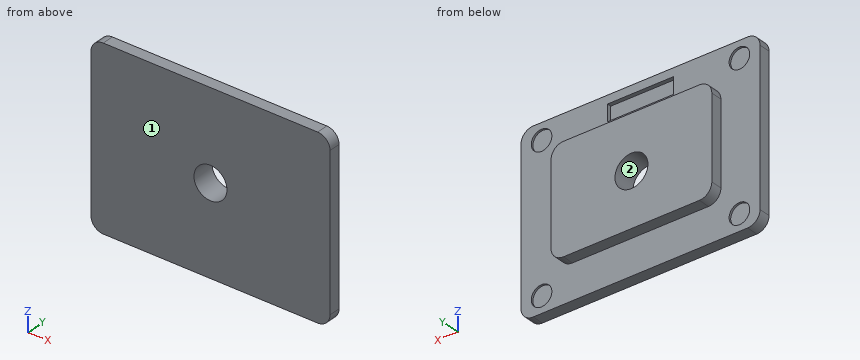
```python
from build123d import *

# Parameters (mm, degrees)
SKETCH3_W                      = 73.66
SKETCH3_H                      = 54.61
EXTRUDED_LOWER_PLATE_DEPTH     = 3.556
SKETCH4_W                      = 49.53
SKETCH4_H                      = 33.02
EXTRUDED_UPPER_PLATE_DEPTH     = 3.556
PLATE_CORNER_FILLET_R          = 3.81
F_0_4D_HOLE_D                  = 10.16
SKETCH9_W                      = 20.32
SKETCH9_H                      = 5.08
EXTRUDED_RECTANGULAR_CUT_DEPTH = 1.27
F_4X_0_25D_PINS_D              = 6.35
F_4X_0_25D_PINS_DEPTH          = 0.635


with BuildPart() as part:
    # Sketch3 → Extruded Lower Plate (new body)
    with BuildSketch(Plane(origin=(0, 0, 0), x_dir=(1, 0, 0), z_dir=(0, 1, 0))):
        Rectangle(SKETCH3_W, SKETCH3_H)
    extrude(amount=EXTRUDED_LOWER_PLATE_DEPTH)

    # Sketch4 → Extruded Upper Plate (add)
    with BuildSketch(Plane(origin=(0, 3.556, 0), x_dir=(1, 0, 0), z_dir=(0, 1, 0))):
        Rectangle(SKETCH4_W, SKETCH4_H)
    extrude(amount=EXTRUDED_UPPER_PLATE_DEPTH)

    # Plate Corner Fillet
    plate_corner_fillet_edges = [part.edges().sort_by_distance(p)[0] for p in [
        (24.765, 5.334, -16.51),
        (-24.765, 5.334, -16.51),
        (-24.765, 5.334, 16.51),
        (24.765, 5.334, 16.51),
        (-36.83, 1.778, -27.305),
        (36.83, 1.778, -27.305),
        (36.83, 1.778, 27.305),
        (-36.83, 1.778, 27.305),
    ]]
    fillet(plate_corner_fillet_edges, radius=PLATE_CORNER_FILLET_R)

    # 0.4D Hole (through all)
    with Locations(Plane(origin=(0, 7.112, 0), x_dir=(1, 0, 0), z_dir=(0, 1, 0))):
        with Locations((0, 0)):
            Hole(F_0_4D_HOLE_D / 2)

    # Sketch9 → Extruded Rectangular Cut (cut)
    with BuildSketch(Plane(origin=(0, 3.556, 0), x_dir=(1, 0, 0), z_dir=(0, 1, 0))):
        with Locations((0, -22.225)):
            Rectangle(SKETCH9_W, SKETCH9_H)
    extrude(amount=-EXTRUDED_RECTANGULAR_CUT_DEPTH, mode=Mode.SUBTRACT)

    # 4X 0.25D Pins
    with Locations(Plane(origin=(0, 3.556, 0), x_dir=(1, 0, 0), z_dir=(0, 1, 0))):
        with Locations((-30.48, -22.225), (-30.48, 22.225), (30.48, 22.225), (30.48, -22.225)):
            Hole(F_4X_0_25D_PINS_D / 2, depth=F_4X_0_25D_PINS_DEPTH)


solid = part.part
```
Geometry: final body of the model. Coordinates: model frame, mm. Face numbers are marked on the shaded views. Round coordinates to 2 decimals unless told otherwise and drop trailing zeros. Loops run counter-clockwise (first coordinate to the right, second up) from the corner with the lowest first, then second, coordinate; pieces in that order, holes last. Notation, with made-up numbers: (73.25, 40.25) -> (99.25, 40.25) arc R12 ccw to (99.25, 62.25) -> close; hole circle Ø11 at (-35, 15.25). An arc over 180 degrees is marked (long way). Write each question's results on one line, items separated by ' | '.
Item 1: Cut plane B-B on y = 5.75. Return the cut outline in (x, z) (3 decimals), and give its area (3 significant figures).
Answers below:
outline: (-24.765, -12.7) arc R3.81 ccw to (-20.955, -16.51) -> (20.955, -16.51) arc R3.81 ccw to (24.765, -12.7) -> (24.765, 12.7) arc R3.81 ccw to (20.955, 16.51) -> (-20.955, 16.51) arc R3.81 ccw to (-24.765, 12.7) -> close; hole circle Ø10.16 at (0, 0) | area: 1,540 mm²
Item 2: Line query: probe 1 along Z at (x, y) = (-30.48, 3.25) (3 decimals); probe 2 along Z at (x, y) = (0, 2.25) (3 decimals); probe 3 along Z at (x, y) = (0, 4). Output: solid intervals per line, ascending. Write a range as [from, to].
Answers below:
probe 1: z = [-27.305, -25.4], [-19.05, 19.05], [25.4, 27.305] | probe 2: z = [-27.305, -5.08], [5.08, 27.305] | probe 3: z = [-16.51, -5.08], [5.08, 16.51]
Item 3: Cut plane A-A on z = 0. Return the cut outline in (x, y) (3 decimals).
Answers below:
outline: (-36.83, 0) -> (-5.08, 0) -> (-5.08, 7.112) -> (-24.765, 7.112) -> (-24.765, 3.556) -> (-36.83, 3.556) -> close; (5.08, 0) -> (36.83, 0) -> (36.83, 3.556) -> (24.765, 3.556) -> (24.765, 7.112) -> (5.08, 7.112) -> close
Item 4: Pull-direction query (X, two-part tool) for the marked faces 1 and 2; classes: pulls with the +X half, pulls with the -X half, needs draft (parallel to the pull), parting line crosses it, or undercut.
Answers below:
face 1: needs draft | face 2: undercut
Item 5: Cut plane C-C on x = 0. Return the cut outline in (y, z) (3 decimals), and give its area (3 significant figures).
Answers below:
outline: (0, -27.305) -> (3.556, -27.305) -> (3.556, -16.51) -> (7.112, -16.51) -> (7.112, -5.08) -> (0, -5.08) -> close; (0, 5.08) -> (7.112, 5.08) -> (7.112, 16.51) -> (3.556, 16.51) -> (3.556, 19.685) -> (2.286, 19.685) -> (2.286, 24.765) -> (3.556, 24.765) -> (3.556, 27.305) -> (0, 27.305) -> close | area: 233 mm²
Item 6: Cut plane D-D on x = -16. Return the cut outline in (y, z) (3 decimals), and give its area (3 significant figures).
Answers below:
outline: (0, -27.305) -> (3.556, -27.305) -> (3.556, -16.51) -> (7.112, -16.51) -> (7.112, 16.51) -> (3.556, 16.51) -> (3.556, 27.305) -> (0, 27.305) -> close | area: 312 mm²
Item 7: Pin query (flat end, axial travel): pin 1 Ø3 at (x, y) = (-4.5, 6) entering from +Z; pin 2 Ø1.9 at (x, z) = (-29.5, 24) entering from +Y; pin 3 Ø5 at (x, z) = (31, 21) entering from +Y. Return the tip coordinate at first contact, or that it passes through.
Answers below:
pin 1: stops at z = 16.51 | pin 2: stops at y = 2.92 | pin 3: stops at y = 3.56
